Source: three-view drawing plus pictorial views. Frame: mm from the lowest corner of the part. Coordinates: 2 decimals unless noted, no trailing zeros. Write each loop counter-clockwise with the first axis right and the second up, starting at its lowest first coordinate (ties: lowest second). Pieces come first, ordered by that corner, then holes. Notation, with made-up numbers: (22, -39) -> (34, -39) arc R10 ccw to (34, -22) -> close; hole circle Ø11 at (-32.75, 60). An arc over 180 degrees is marked (long way). One line per question, with ' | ' between items. Start each with the question number.
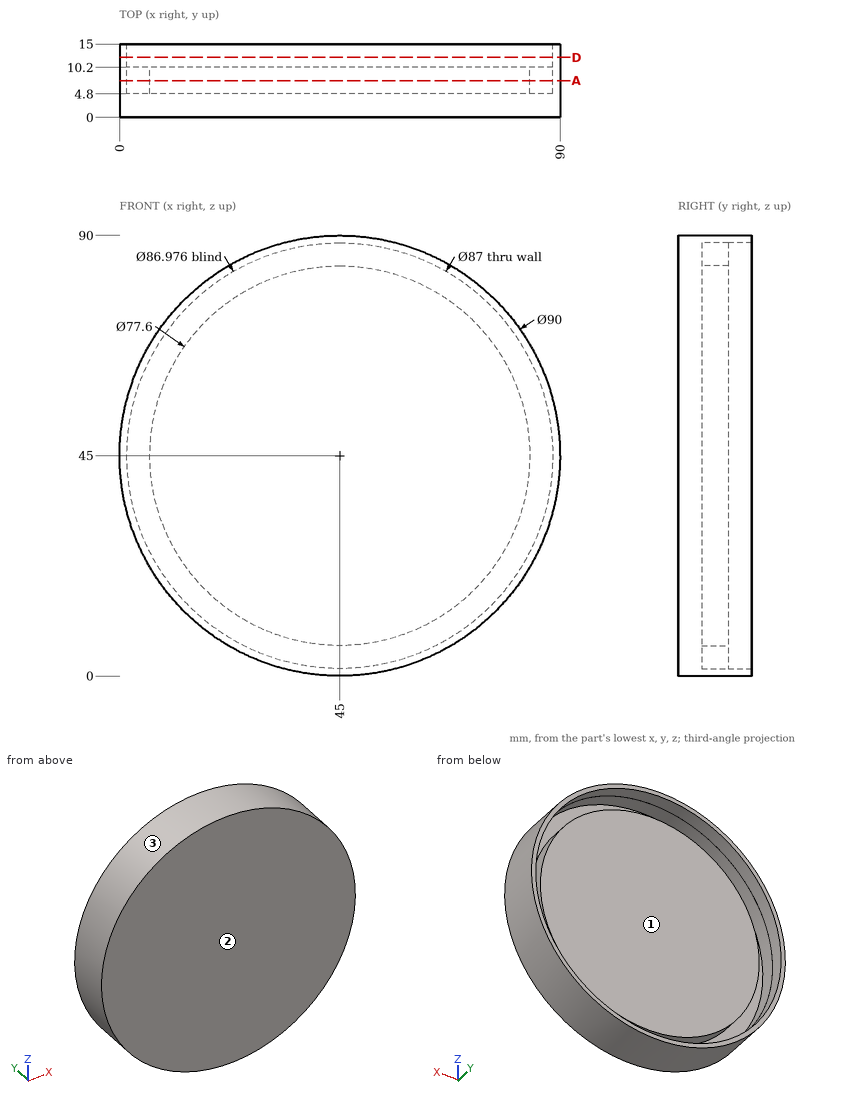
1) First-contact query: P1, Ø1.5, axis at x = 76, z = 18.5, coming from the -Y side; P2, Ø3, axis at y = 11.5, z = 41.5, coming from the -X side; P3, Ø2, axis at x = 22.5, z = 44, coming from the +Y side; P4, Ø2, axis at y = 10, z = 13.5, coming from the -X side. Flat tips, straight axial feed; report the tip coordinate or a pass-through.
2) Ray query, line 1 (X direction, y = 7.75, z = 32.5); line 2 (Z direction, x = 37.5, y = 5); line 3 (X direction, y = 9.5, z = 69.5). Return the intervals inside material, ascending.
3) Section D-D, the plane y = 12.25. Return loops of the section in (x, z).
4) Pull-direction query (X, two-part tool) for the marked faces 1, 2 and 3; classes: released by +X, released by -X, zero draft, split by the parting line, or undercut.
5) Section A-A, the plane y = 7.5. Return loops of the section in (x, z).
Answer block:
1) P1: stops at y = 0 | P2: stops at x = 0.04 | P3: stops at y = 10.2 | P4: stops at x = 11.91
2) line 1: x = 1.77 to 3.35, 8.27 to 81.73, 86.65 to 88.23 | line 2: z = 0.63 to 2.16, 6.93 to 83.07, 87.84 to 89.37 | line 3: x = 7.25 to 9.07, 14.91 to 75.09, 80.93 to 82.75
3) outline: circle Ø90 at (45, 45); hole circle Ø87 at (45, 45)
4) face 1: undercut | face 2: zero draft | face 3: split by the parting line
5) outline: circle Ø90 at (45, 45); circle Ø77.6 at (45, 45); hole circle Ø86.98 at (45, 45)
